```python
from build123d import *

# Parameters (mm, degrees)
SKETCH1_W           = 254
SKETCH1_H           = 317.5
BOSS_EXTRUDE1_DEPTH = 6.35
SKETCH2_W           = 25.4
SKETCH2_H           = 6.35
CUT_EXTRUDE1_DEPTH  = 6.35
LPATTERN1_COUNT     = 5
LPATTERN1_PITCH     = 50.8


with BuildPart() as part:
    # Sketch1 → Boss-Extrude1 (new body)
    with BuildSketch(Plane.XY):
        with Locations((127, 158.75)):
            Rectangle(SKETCH1_W, SKETCH1_H)
    extrude(amount=BOSS_EXTRUDE1_DEPTH)

    # Sketch2 → Cut-Extrude1 (cut)
    with BuildSketch(Plane.XY):
        with Locations((38.1, 314.325)):
            Rectangle(SKETCH2_W, SKETCH2_H)
    cut_extrude1 = extrude(amount=CUT_EXTRUDE1_DEPTH, mode=Mode.SUBTRACT)

    # LPattern1: Cut-Extrude1 ×5
    with Locations(*[(i * LPATTERN1_PITCH, 0, 0) for i in range(1, LPATTERN1_COUNT)]):
        add(cut_extrude1, mode=Mode.SUBTRACT)


solid = part.part
```
The listing builds one solid part. Answer for the finished solid, in the listing's coordinates (mm). A direction names the side the tool comes from. Give positions to 0.01 mm unless a question says otherwise; leave off trailing zeros. Loops run counter-clockwise (first coordinate to the right, second up) from the corner with the lowest first, then second, coordinate; pieces in that order, holes last. Notation, with made-up numbers: M 59,-37 L 110,-37 A22 cw 110,-16 Z; hole C 83,62 d4. An arc over 180 degrees is marked long. One line per item, written item: value.
1. Each of these flat-tipped pins is pushed along its axis until it touches: P1, Ø3, axis at y = 313.5, z = 4, coming from the +X side; P2, Ø1.9, axis at x = 189.5, z = 3, coming from the +Y side. Where does it stop, or does it pass through?
Found:
P1: x = 228.6
P2: y = 311.15
2. Section A-A on x = 139 is taken. Determine the outline of the cut face in (y, z), plus the area to 3 significant figures.
Found:
outline: M 0,0 L 311.15,0 L 311.15,6.35 L 0,6.35 Z
area: 1,980 mm^2
3. For faces 1 (the face through (241, 311.15, 3)), 2 (the face through (254, 153, 3)), 3 (the face through (190, 311.15, 3)), determine the directions among +Z, -Z, +X, -X, +Y, -Y from which every point of the face is accessible in a straight line to the end or side of a thin tool.
Found:
face 1: +Z, -Z, +X, +Y
face 2: +Z, -Z, +X, +Y, -Y
face 3: +Z, -Z, +Y
4. For a pull along X with two mould halves and no side action, classify faces 4 (the face through (228.6, 314, 3)), 5 (the face through (140, 311.15, 3)), 6 (the face through (125, 161, 0)) as pulls with the +X half, pulls with the -X half, needs draft (parallel to the pull), parting line crosses it, or undercut.
Found:
face 4: pulls with the +X half
face 5: undercut
face 6: needs draft
5. Find the intervals of material crossed by probe 1 along Y at (x, z) = (191, 3.25), in increasing order.
Found:
probe 1: 0 to 311.15
